Could you check a few things on this model? Use its own coordinates, in mm. A direction names the side the tool comes from. Give positions to 0.01 mm unless a question says otherwise; leave off trailing zeros. Write each loop counter-clockwise with the first axis right and the second up, starting at its lowest first coordinate (ties: lowest second). Pieces come first, ordered by that corner, then holes. Notation, with made-up numbers: M 50,2 L 79,2 A25 ccw 79,21 Z; hole C 68,27 d8. An arc over 180 degrees is marked long. One line per item, written item: value.
```python
from build123d import *

# Parameters (mm, degrees)
BOSS_EXTRUDE1_DEPTH      = 8
BOSS_EXTRUDE2_DEPTH      = 46.583974855
BOSS_EXTRUDE2_DEPTH_BACK = 46.58397486
SKETCH4_R                = 3.3
CUT_EXTRUDE1_DEPTH       = 32.2
CUT_EXTRUDE1_DEPTH_BACK  = 32.2
SKETCH5_R                = 3.3
SKETCH6_W                = 40
SKETCH6_H                = 3
BOSS_EXTRUDE3_DEPTH      = 40
SKETCH7_R                = 2
CUT_EXTRUDE2_DEPTH       = 233.497849452
SKETCH8_W                = 20
SKETCH8_H                = 3
CUT_EXTRUDE3_DEPTH       = 30
SKETCH9_R                = 2
CUT_EXTRUDE4_DEPTH       = 233.570419443
FILLET1_R                = 20
SKETCH10_R               = 1.5
CUT_EXTRUDE5_DEPTH       = 10
SCALE1_SCALE             = 1.5
SCALE2_SCALE             = 0.8
SKETCH12_R               = 1.8
BOSS_EXTRUDE4_DEPTH      = 9.6
SKETCH13_R               = 2
SKETCH13_R_2             = 2.5
CUT_EXTRUDE6_DEPTH       = 262.790915701
BOSS_EXTRUDE5_REACH      = 322.905
SKETCH14_R               = 4.250728377
SKETCH14_R_2             = 3
SKETCH15_W               = 77.28
SKETCH15_H               = 12
CUT_EXTRUDE7_DEPTH       = 262.790915701
BOSS_EXTRUDE6_START      = -3.6
SKETCH16_R               = 2.5
BOSS_EXTRUDE6_DEPTH      = 3.6
SKETCH17_R               = 2.5
CUT_EXTRUDE8_DEPTH       = 262.698077073


with BuildPart() as part:
    # Sketch1 → Boss-Extrude1 (new body)
    with BuildSketch(Plane(origin=(0, 0, 0), x_dir=(1, 0, 0), z_dir=(0, 1, 0))):
        Polygon((-120, -37.5), (-120, -75), (0, -75), (0, 75), (-120, 75), (-120, 37.5), (-220, 37.5), (-220, -37.5), align=None)
    extrude(amount=BOSS_EXTRUDE1_DEPTH)

    # Sketch4 → Boss-Extrude2 (add, two sides: drawn at the far end of the back side and taken through both)
    # profile 1 of 2: a face of its own
    with BuildSketch(Plane.ZY.offset(170).offset(-BOSS_EXTRUDE2_DEPTH_BACK)):
        with BuildLine():
            Line((37.5, 8), (43.5, 8))
            ThreePointArc((43.5, 8), (47.5, 4), (43.5, 0))
            Line((43.5, 0), (37.5, 0))
            Line((37.5, 0), (37.5, 8))
        make_face()
        with Locations((43.5, 4)):
            Circle(SKETCH4_R, mode=Mode.SUBTRACT)
    # profile 2 of 2: a face of its own
    with BuildSketch(Plane.ZY.offset(170).offset(-BOSS_EXTRUDE2_DEPTH_BACK)):
        with BuildLine():
            Line((-37.5, 0), (-43.5, 0))
            ThreePointArc((-43.5, 0), (-47.5, 4), (-43.5, 8))
            Line((-43.5, 8), (-37.5, 8))
            Line((-37.5, 8), (-37.5, 0))
        make_face()
        with Locations((-43.5, 4)):
            Circle(SKETCH4_R, mode=Mode.SUBTRACT)
    extrude(amount=BOSS_EXTRUDE2_DEPTH + BOSS_EXTRUDE2_DEPTH_BACK)

    # Sketch5 → Cut-Extrude1 (cut, two sides: drawn at the far end of the back side and taken through both)
    # profile 1 of 2: a face of its own
    with BuildSketch(Plane.ZY.offset(170).offset(-CUT_EXTRUDE1_DEPTH_BACK)):
        with BuildLine():
            Line((-43.5, 8), (-37.5, 8))
            Line((-37.5, 8), (-37.5, 0))
            Line((-37.5, 0), (-43.5, 0))
            ThreePointArc((-43.5, 0), (-47.5, 4), (-43.5, 8))
        make_face()
        with Locations((-43.5, 4)):
            Circle(SKETCH5_R, mode=Mode.SUBTRACT)
    # profile 2 of 2: a face of its own
    with BuildSketch(Plane.ZY.offset(170).offset(-CUT_EXTRUDE1_DEPTH_BACK)):
        with BuildLine():
            Line((37.5, 0), (43.5, 0))
            ThreePointArc((43.5, 0), (47.5, 4), (43.5, 8))
            Line((43.5, 8), (37.5, 8))
            Line((37.5, 8), (37.5, 0))
        make_face()
        with Locations((43.5, 4)):
            Circle(SKETCH5_R, mode=Mode.SUBTRACT)
    extrude(amount=CUT_EXTRUDE1_DEPTH + CUT_EXTRUDE1_DEPTH_BACK, mode=Mode.SUBTRACT)

    # Sketch6 → Boss-Extrude3 (add)
    with BuildSketch(Plane(origin=(0, 0, 0), x_dir=(0, 0, -1), z_dir=(1, 0, 0))):
        with Locations((0, 4)):
            Rectangle(SKETCH6_W, SKETCH6_H)
    extrude(amount=BOSS_EXTRUDE3_DEPTH)

    # Sketch7 → Cut-Extrude2 (cut, through all)
    with BuildSketch(Plane(origin=(0, 5.5, 0), x_dir=(1, 0, 0), z_dir=(0, 1, 0))):
        with Locations(Location((32.75, 0, 0), (0, 0, 270))):
            Circle(SKETCH7_R)
    extrude(amount=-CUT_EXTRUDE2_DEPTH, mode=Mode.SUBTRACT)

    # Sketch8 → Cut-Extrude3 (cut)
    with BuildSketch(Plane(origin=(0, 0, 0), x_dir=(0, 0, -1), z_dir=(1, 0, 0))):
        with Locations((-50, 4)):
            Rectangle(SKETCH8_W, SKETCH8_H)
        with Locations((50, 4)):
            Rectangle(SKETCH8_W, SKETCH8_H)
    extrude(amount=-CUT_EXTRUDE3_DEPTH, mode=Mode.SUBTRACT)

    # Sketch9 → Cut-Extrude4 (cut, through all)
    with BuildSketch(Plane(origin=(0, 8, 0), x_dir=(1, 0, 0), z_dir=(0, 1, 0))):
        with Locations(Location((-22.5, -50, 0), (0, 0, 270))):
            Circle(SKETCH9_R)
        with Locations(Location((-22.5, 50, 0), (0, 0, 90))):
            Circle(SKETCH9_R)
    extrude(amount=-CUT_EXTRUDE4_DEPTH, mode=Mode.SUBTRACT)

    # Fillet1
    # the kernel refuses this fillet: 20 mm, written as the material it takes off along each edge
    with BuildSketch(Plane(origin=(-220, -27.947694226, 37.5), x_dir=(1, 0, 0), z_dir=(0, 1, 0))) as fillet1_piece_1:
        with BuildLine():
            CenterArc((20, 11.17907769), FILLET1_R, 180, 33.98348272)
            Line((0, 11.17907769), (-0.4, 11.17907769))
            Line((-0.4, 11.17907769), (-0.4, 0))
            Line((-0.4, 0), (0, -0.4))
            ThreePointArc((0, -0.4), (1.708012572, -0.4), (3.084345648, -0.223581554))
            Line((3.084345648, -0.223581554), (3.416025145, 0))
        make_face()
    extrude(amount=63.895388452, mode=Mode.SUBTRACT)
    with BuildSketch(Plane(origin=(-220, -27.947694226, -37.5), x_dir=(0, 0, 1), z_dir=(0, 1, 0))) as fillet1_piece_2:
        with BuildLine():
            CenterArc((11.17907769, 20), FILLET1_R, 236.01651728, 33.98348272)
            Line((0, 3.416025145), (-0.223581554, 3.084345648))
            ThreePointArc((-0.223581554, 3.084345648), (-0.4, 1.708012572), (-0.4, 0))
            Line((-0.4, 0), (0, -0.4))
            Line((0, -0.4), (11.17907769, -0.4))
            Line((11.17907769, -0.4), (11.17907769, 0))
        make_face()
    extrude(amount=63.895388452, mode=Mode.SUBTRACT)
    with BuildSketch(Plane(origin=(-120, -50, -75), x_dir=(1, 0, 0), z_dir=(0, 1, 0)), Plane(origin=(-120, -50, 75), x_dir=(0, 0, -1), z_dir=(0, 1, 0))) as fillet1_piece_3:
        with BuildLine():
            CenterArc((FILLET1_R, -FILLET1_R), FILLET1_R, 90, 90)
            Line((0, -FILLET1_R), (-FILLET1_R * 0.02, -FILLET1_R))
            Line((-FILLET1_R * 0.02, -FILLET1_R), (-FILLET1_R * 0.02, FILLET1_R * 0.02))
            Line((-FILLET1_R * 0.02, FILLET1_R * 0.02), (FILLET1_R, FILLET1_R * 0.02))
            Line((FILLET1_R, FILLET1_R * 0.02), (FILLET1_R, 0))
        make_face()
    extrude(amount=108, mode=Mode.SUBTRACT)

    # Sketch10 → Cut-Extrude5 (cut)
    with BuildSketch(Plane(origin=(0, 8, 0), x_dir=(1, 0, 0), z_dir=(0, 1, 0))):
        with Locations(Location((-25, 72.5, 0), (0, 0, 270))):
            Circle(SKETCH10_R)
        with Locations(Location((-75, 72.5, 0), (0, 0, 270))):
            Circle(SKETCH10_R)
        with Locations(Location((-25, -72.5, 0), (0, 0, 270))):
            Circle(SKETCH10_R)
        with Locations(Location((-75, -72.5, 0), (0, 0, 270))):
            Circle(SKETCH10_R)
    extrude(amount=-CUT_EXTRUDE5_DEPTH, mode=Mode.SUBTRACT)


with BuildPart() as part_1:
    # Scale1: scaled about (-91.766272815, 4, 0)
    add(part.part.scale(SCALE1_SCALE).moved(Location((45.883136407, -2, 0))))


with BuildPart() as part_2:
    # Scale2: scaled about (-91.766272815, 4, 0)
    add(part_1.part.scale(SCALE2_SCALE).moved(Location((-18.353254563, 0.8, 0))))

    # Sketch12 → Boss-Extrude4 (add, through all)
    with BuildSketch(Plane(origin=(0, 8.8, 0), x_dir=(1, 0, 0), z_dir=(0, 1, 0))):
        with Locations((-71.646745437, 87)):
            Circle(SKETCH12_R)
        with Locations((-11.646745437, 87)):
            Circle(SKETCH12_R)
        with Locations((-11.646745437, -87)):
            Circle(SKETCH12_R)
        with Locations((-71.646745437, -87)):
            Circle(SKETCH12_R)
    extrude(amount=-BOSS_EXTRUDE4_DEPTH)

    # Sketch13 → Cut-Extrude6 (cut, through all)
    with BuildSketch(Plane.XZ.offset(0.8)):
        with Locations(Location((-71.646745437, 86.7, 0), (0, 0, 270))):
            Circle(SKETCH13_R)
        with Locations(Location((-11.646745437, 86.7, 0), (0, 0, 90))):
            Circle(SKETCH13_R)
        with Locations(Location((-11.646745437, -86.7, 0), (0, 0, 270))):
            Circle(SKETCH13_R)
        with Locations(Location((-71.646745437, -86.7, 0), (0, 0, 90))):
            Circle(SKETCH13_R)
        with Locations(Location((-8.646745437, 60, 0), (0, 0, 270))):
            Circle(SKETCH13_R_2)
        with Locations(Location((57.653254563, 0, 0), (0, 0, 270))):
            Circle(SKETCH13_R_2)
        with Locations(Location((-8.646745437, -60, 0), (0, 0, 270))):
            Circle(SKETCH13_R_2)
    extrude(amount=-CUT_EXTRUDE6_DEPTH, mode=Mode.SUBTRACT)

    # Boss-Extrude5: up to this face of the body (flat: up to its plane)
    boss_extrude5_end = Plane(part_2.part.faces().sort_by_distance((-129.745975605, 8.646325018, -48.6))[0])
    # Sketch14 → Boss-Extrude5 (add, up to the picked face)
    with BuildSketch(Plane.ZY.offset(241.547515263), mode=Mode.PRIVATE) as boss_extrude5_sk1:
        with Locations((-52.2, 4)):
            Circle(SKETCH14_R)
        with Locations((-52.2, 4)):
            Circle(SKETCH14_R_2, mode=Mode.SUBTRACT)
    boss_extrude5_tool1 = split(extrude(boss_extrude5_sk1.sketch, amount=-BOSS_EXTRUDE5_REACH, mode=Mode.PRIVATE), bisect_by=boss_extrude5_end, keep=Keep.BOTH, mode=Mode.PRIVATE)
    # Sketch14 → Boss-Extrude5 (add, up to the picked face)
    with BuildSketch(Plane.ZY.offset(241.547515263), mode=Mode.PRIVATE) as boss_extrude5_sk2:
        with Locations(Location((52.2, 4, 0), (0, 0, 180))):
            Circle(SKETCH14_R)
        with Locations(Location((52.2, 4, 0), (0, 0, 180))):
            Circle(SKETCH14_R_2, mode=Mode.SUBTRACT)
    boss_extrude5_tool2 = split(extrude(boss_extrude5_sk2.sketch, amount=-BOSS_EXTRUDE5_REACH, mode=Mode.PRIVATE), bisect_by=boss_extrude5_end, keep=Keep.BOTH, mode=Mode.PRIVATE)
    add(boss_extrude5_tool1.solids().sort_by(Axis((-241.547515, 4, -56.3305), (1, 0, 0)))[0])
    add(boss_extrude5_tool2.solids().sort_by(Axis((-241.547515, 4, 56.3305), (1, 0, 0)))[0])

    # Sketch15 → Cut-Extrude7 (cut, through all)
    with BuildSketch(Plane(origin=(0, 8.8, 0), x_dir=(1, 0, 0), z_dir=(0, 1, 0))):
        with Locations((-185.646745437, 51)):
            Rectangle(SKETCH15_W, SKETCH15_H)
        with Locations((-185.646745437, -51)):
            Rectangle(SKETCH15_W, SKETCH15_H)
    extrude(amount=-CUT_EXTRUDE7_DEPTH, mode=Mode.SUBTRACT)

    # Sketch16 → Boss-Extrude6 (add)
    with BuildSketch(Plane(origin=(0, 5.8, 0), x_dir=(1, 0, 0), z_dir=(0, 1, 0)).offset(BOSS_EXTRUDE6_START)):
        with Locations((57.653254563, 0)):
            Circle(SKETCH16_R)
    extrude(amount=BOSS_EXTRUDE6_DEPTH)

    # Sketch17 → Cut-Extrude8 (cut, through all)
    with BuildSketch(Plane(origin=(0, 5.8, 0), x_dir=(1, 0, 0), z_dir=(0, 1, 0))):
        with Locations(Location((57.353254563, 0, 0), (0, 0, 270))):
            Circle(SKETCH17_R)
    extrude(amount=-CUT_EXTRUDE8_DEPTH, mode=Mode.SUBTRACT)


solid = part_2.part
```
1) Please list where these lines run through material, in increasing order: L1, parallel to X at y = 4.5, z = 46; L2, parallel to X at y = 4.4, z = 0; L3, parallel to X at y = 0.6, z = -60. Write a range as from..to.
Outcome:
L1: x = -241.55..-224.29, -147.01..-129.75, -125.65..18.35
L2: x = -245.65..54.85, 59.85..66.35
L3: x = -125.65..-11.15, -6.15..18.35
2) On a 3-axis mill with a long thin cutter (end or side, diameter ignored), from which of +Z, -Z, +X, -X, +Y, -Y can I reach the whole of each face in a straight line? I mean faces 1 (the face through (-125.647, 4, 55)), 2 (the face through (-241.548, 4, -48)), 3 (the face through (-233.04, 4.9, -49.34)), 4 (the face through (-224.287, 4, -48)), 5 (the face through (42, 2.2, 0)). Say none if no direction works.
Outcome:
face 1: +Z, +Y, -Y
face 2: -Z, -X, +Y, -Y
face 3: -X
face 4: -Z, +Y, -Y
face 5: +Z, -Z, +X, -Y
3) We'd pull the mould along X, two halves only. Please class faces 6 (the face through (-125.647, 4, -56)), 7 (the face through (1, 5.8, 60)), 8 (the face through (-241.548, 4, 48)): pulls with the +X half, pulls with the -X half, needs draft (parallel to the pull), parting line crosses it, or undercut.
Outcome:
face 6: undercut
face 7: needs draft
face 8: pulls with the -X half
4) If we section it at A-A, the plane x = -134.5: Write out the boundary of the cut face in (y, z).
Outcome:
outline: M -0.8,-52.2 A4.8 ccw 8.8,-52.2 L 8.8,52.2 A4.8 ccw -0.8,52.2 Z; hole C 4,-52.2 d6; hole C 4,52.2 d6
5) If we section it at C-C, the plane z = 36: Write out the boundary of the cut face in (x, y).
Outcome:
outline: M -245.24,-0.8 L 18.35,-0.8 L 18.35,8.8 L -245.24,8.8 Z
6) If we section it at B-B, the plane y = 4: Give the number of separate pieces and of enclosed holes in the cut face, then the cut area to 3 significant figures.
Outcome:
separate pieces: 5
enclosed holes: 5
area: 37,400 mm^2
7) If we section it at D-D, the plane x = 25.5: Write out the boundary of the cut face in (y, z), then the cut area to 3 significant figures.
Outcome:
outline: M 2.2,-24 L 5.8,-24 L 5.8,24 L 2.2,24 Z
area: 173 mm^2
8) I'm going to push flat-ended pins straight in: pin 1 (1.1 mm diameter, centred on x = 47.5, y = 4, fed in from -Z); pin 2 (3 mm diameter, centred on x = -8.65, z = -60, fed in from -Y); pin 3 (3 mm diameter, centred on x = 37, y = 4.5, fed in from +Z); pin 4 (3 mm diameter, centred on x = -154, y = 0, fed in from +Z). Where does each tip first touch, or does it pass through?
Outcome:
pin 1: stops at z = -24
pin 2: passes through
pin 3: stops at z = 24
pin 4: stops at z = 45
